from build123d import *

# Parameters (mm, degrees)
F0_R     = 2.55
F1_DEPTH = 7
F3_DEPTH = 2.5
F6_DEPTH = 1.2


with BuildPart() as f1:
    # F0 (on Top) → F1 (new body)
    with BuildSketch(Plane.XY):
        with BuildLine():
            ThreePointArc((-22.0288725662, 15.0277765828), (-23.9870436526, 16.827971802), (-24.9929573966, 19.2903434982))
            ThreePointArc((-24.9929573966, 19.2903434982), (-34.8, 23.9023011445), (-35.7094488189, 13.1031742908))
            ThreePointArc((-35.7094488189, 13.1031742908), (-34.0799292484, 11.0008415863), (-33.5, 8.404918071))
            Line((-33.5, 8.404918071), (-33.5, -8.404918071))
            ThreePointArc((-33.5, -8.404918071), (-34.0799292484, -11.0008415863), (-35.7094488189, -13.1031742908))
            ThreePointArc((-35.7094488189, -13.1031742908), (-34.8, -23.9023011445), (-24.9929573966, -19.2903434982))
            ThreePointArc((-24.9929573966, -19.2903434982), (-23.9870430876, -16.8279709896), (-22.0288708522, -15.0277755932))
            Line((-22.0288708522, -15.0277755932), (-17.348076829, -12.3253179039))
            ThreePointArc((-17.348076829, -12.3253179039), (-16.6160260214, -9.5932670963), (-19.348076829, -8.8612162887))
            Line((-19.348076829, -8.8612162887), (-24.0288708522, -11.5636739781))
            ThreePointArc((-24.0288708522, -11.5636739781), (-27.6762899984, -11.5636754624), (-29.5, -8.404918071))
            Line((-29.5, -8.404918071), (-29.5, 8.404918071))
            ThreePointArc((-29.5, 8.404918071), (-27.6762908554, 11.5636749676), (-24.0288725662, 11.5636749676))
            Line((-24.0288725662, 11.5636749676), (-9.4711274338, 3.1587568967))
            ThreePointArc((-9.4711274338, 3.1587568967), (-7.6474182892, -9.615e-07), (-9.4711290992, -3.1587578582))
            Line((-9.4711290992, -3.1587578582), (-14.1519236685, -5.8612158628))
            ThreePointArc((-14.1519236685, -5.8612158628), (-14.8839746302, -8.5932681071), (-12.1519222705, -9.3253186383))
            Line((-12.1519222705, -9.3253186383), (-7.4711290992, -6.6228594733))
            ThreePointArc((-7.4711290992, -6.6228594733), (-4.9330280571, -5.8271302964), (-2.2975937845, -6.1871692074))
            ThreePointArc((-2.2975937845, -6.1871692074), (6.6, 0), (-2.2975937845, 6.1871692074))
            ThreePointArc((-2.2975937845, 6.1871692074), (-4.933027099, 5.8271302157), (-7.4711274338, 6.6228585118))
            Line((-7.4711274338, 6.6228585118), (-22.0288725662, 15.0277765828))
        make_face()
        with Locations((-31.5, -18.1865334795)):
            Circle(F0_R, mode=Mode.SUBTRACT)
        with Locations((-31.5, 18.1865334795)):
            Circle(F0_R, mode=Mode.SUBTRACT)
        Circle(F0_R, mode=Mode.SUBTRACT)
    extrude(amount=F1_DEPTH)

    # F2 (on face) → F3 (cut)
    with BuildSketch(Plane.XY.offset(7)):
        Polygon((-27.5, 15.8771324027), (-27.5, 20.4959345562), (-31.5, 22.805335633), (-35.5, 20.4959345562), (-35.5, 15.8771324027), (-31.5, 13.567731326), align=None)
        Polygon((-27.5, -20.4959345562), (-27.5, -15.8771324027), (-31.5, -13.567731326), (-35.5, -15.8771324027), (-35.5, -20.4959345562), (-31.5, -22.805335633), align=None)
        Polygon((-4, 2.3094010768), (-4, -2.3094010768), (0, -4.6188021535), (4, -2.3094010768), (4, 2.3094010768), (0, 4.6188021535), align=None)
    extrude(amount=-F3_DEPTH, mode=Mode.SUBTRACT)

    # F5 (on mid) → F6 (cut, symmetric)
    with BuildSketch(Plane.XY.offset(3.5)):
        with BuildLine():
            Line((-19.348076829, -8.8612162887), (-21.3992959786, -10.045488217))
            ThreePointArc((-21.3992959786, -10.045488217), (-21.0327555807, -12.1432670963), (-19.3992959786, -13.5095898321))
            Line((-19.3992959786, -13.5095898321), (-17.348076829, -12.3253179039))
            ThreePointArc((-17.348076829, -12.3253179039), (-20.0801276365, -11.5932670963), (-19.348076829, -8.8612162887))
        make_face()
        with BuildLine():
            ThreePointArc((-14.1519236685, -5.8612158628), (-11.4198718547, -6.5932667092), (-12.1519222705, -9.3253186383))
            Line((-12.1519222705, -9.3253186383), (-10.1007041172, -8.1410464231))
            ThreePointArc((-10.1007041172, -8.1410464231), (-10.4672447351, -6.043266985), (-12.1007051418, -4.6769442942))
            Line((-12.1007051418, -4.6769442942), (-14.1519236685, -5.8612158628))
        make_face()
    extrude(amount=F6_DEPTH, both=True, mode=Mode.SUBTRACT)


solid = f1.part
Verification items for the finished model (mm, model axes). A direction names the side the tool comes from. Coordinates: 2 decimals unless noted, no trailing zeros. Loops run counter-clockwise (first coordinate to the right, second up) from the corner with the lowest first, then second, coordinate; pieces in that order, holes last. Notation, with made-up numbers: (-15, 66.25) -> (43, 66.25) arc R27 cw to (43, 86.25) -> close; hole circle Ø8 at (68.25, 30). An arc over 180 degrees is marked (long way). Write each question's results on one line, items separated by ' | '.
Item 1: Section check A-A, the plane y = 0. Enter the section's corners in (x, z).
Found:
outline: (-33.5, 0) -> (-29.5, 0) -> (-29.5, 7) -> (-33.5, 7) -> close; (-7.65, 0) -> (-2.55, 0) -> (-2.55, 4.5) -> (-4, 4.5) -> (-4, 7) -> (-7.65, 7) -> close; (2.55, 0) -> (6.6, 0) -> (6.6, 7) -> (4, 7) -> (4, 4.5) -> (2.55, 4.5) -> close
Item 2: Material ranges on L1, parallel to Y at x = -31.5, z = 2.2; L2, parallel to Y at x = 0, z = 2.3; L3, parallel to Y at x = -28.5, z = 4.75, recorded low to high.
Found:
L1: y = -24.79 to -20.74, -15.64 to 15.64, 20.74 to 24.79 | L2: y = -6.6 to -2.55, 2.55 to 6.6 | L3: y = -24.07 to -21.07, -15.3 to -10.91, 10.91 to 15.3, 21.07 to 24.07
Item 3: Tool access check on faces 4 (the face through (-21.048, -12.117, 3.483)), 5 (the face through (-27.63, -11.59, 3.45)), 6 (the face through (-29.472, 21.634, 5.768)). Record the directions out of +Z, -Z, +X, -X, +Y, -Y that give a thin tool (end or side, any length) a straight path to the whole face; none if there is none.
Found:
face 4: none | face 5: +Z, -Z | face 6: +Z
Item 4: Section check C-C, the plane y = 11. Enter the section's corners in (x, z), plus the area to 3 significant figures.
Found:
outline: (-34.08, 0) -> (-28.42, 0) -> (-28.42, 7) -> (-34.08, 7) -> close; (-23.05, 0) -> (-15.05, 0) -> (-15.05, 7) -> (-23.05, 7) -> close | area: 95.6 mm2
Item 5: Gauge pin test, flat ends, axial feed: pin 1 (4 mm diameter, centred on y = 14.5, z = 2, fed in from -X); pin 2 (3.5 mm diameter, centred on y = -3.5, z = 3.5, fed in from -X); pin 3 (1 mm diameter, centred on x = -2.5, z = 5, fed in from -Y). Record the tip position at first contact, or that the pin passes through.
Found:
pin 1: stops at x = -37.88 | pin 2: stops at x = -33.5 | pin 3: stops at y = -6.29
Item 6: Mould release check, pull along Y, two halves, no side actions. Record for faces 1 (the face through (-14.648, 10.766, 3.451)), 2 (the face through (-24.01, -16.86, 3.45)), 3 (the face through (-27.5, -18, 6)): +Y half, -Y half, draft (parallel to the pull), parting line (faces both ways), or undercut.
Found:
face 1: +Y half | face 2: -Y half | face 3: undercut
Item 7: Section check B-B, the plane x = -13.5. Enter the section's corners in (y, z), plus the area to 3 significant figures.
Found:
outline: (-9.56, 0) -> (-5.48, 0) -> (-5.48, 2.3) -> (-5.62, 2.3) -> (-5.62, 4.7) -> (-5.48, 4.7) -> (-5.48, 7) -> (-9.56, 7) -> close; (5.48, 0) -> (10.1, 0) -> (10.1, 7) -> (5.48, 7) -> close | area: 60.5 mm2
Item 8: Section check D-D, the plane z = 6.25. Count the separate pieces of the cut face and the enclosed holes in it, plus the area to 3 significant figures.
Found:
separate pieces: 1 | enclosed holes: 3 | area: 539 mm2
